Study the drawing (mm; zero at the part's minimum x, y, z) and answer. A direction names the side the tool comes from. Coordinates: 2 decimals unless noted, no trailing zeros. Loops run counter-clockwise (first coordinate to the right, second up) from the corner with the lowest first, then second, coordinate; pieces in that order, holes last. Notation, with made-up numbers: (80.5, 35.5) -> (106.5, 35.5) arc R32 ccw to (106.5, 70.5) -> close; hole circle Ø1 at (68, 37). An arc over 180 degrees is marked (long way). Answer as a JSON object with one key per item and string values. Group by question number.
Q1. The part is cut by section B-B on z = 4.75. Write down the section's boundary in (x, y) (1 decimal).
Q2. Determine the mould class of the marked faces 1, 2 and 3 for opening direction X: released by +X, released by -X, zero draft, split by the parting line, or undercut.
Q3. For the marked faces 4, 5 and 6, determine the directions among +Z, -Z, +X, -X, +Y, -Y from which every point of the face is accessible in a straight line to the end or side of a thin tool.
Q4. The part is cut by section C-C on x = 18. Write down the section's boundary in (y, z).
Q5. Straight lines are drawn through the part: line 1 along X through (y, z) = (1.25, 3.5); line 2 along Y through (x, z) = (18.5, 3.5); line 3 along X through (y, z) = (13, 3.5) (1 decimal). For each, find the intervals that lie inside material, in ascending order. Write a range as [from, to].
Q6. The part is cut by section D-D on y = 9.5. Write down the section's boundary in (x, z) (1 decimal).
Q7. The part is cut by section A-A on y = 6.25. Write down the section's boundary in (x, z) (1 decimal).
Q8. Each of these flat-tipped pins is pushed along its axis until it touches: P1, Ø5.5, axis at x = 18.5, z = 6, coming from the -Y side; P2, Ø4, axis at y = 7, z = 5, coming from the +X side; P3, Ø2.5, axis at x = 3.5, z = 9.5, coming from the +Y side. Where does it stop, or does it pass through?
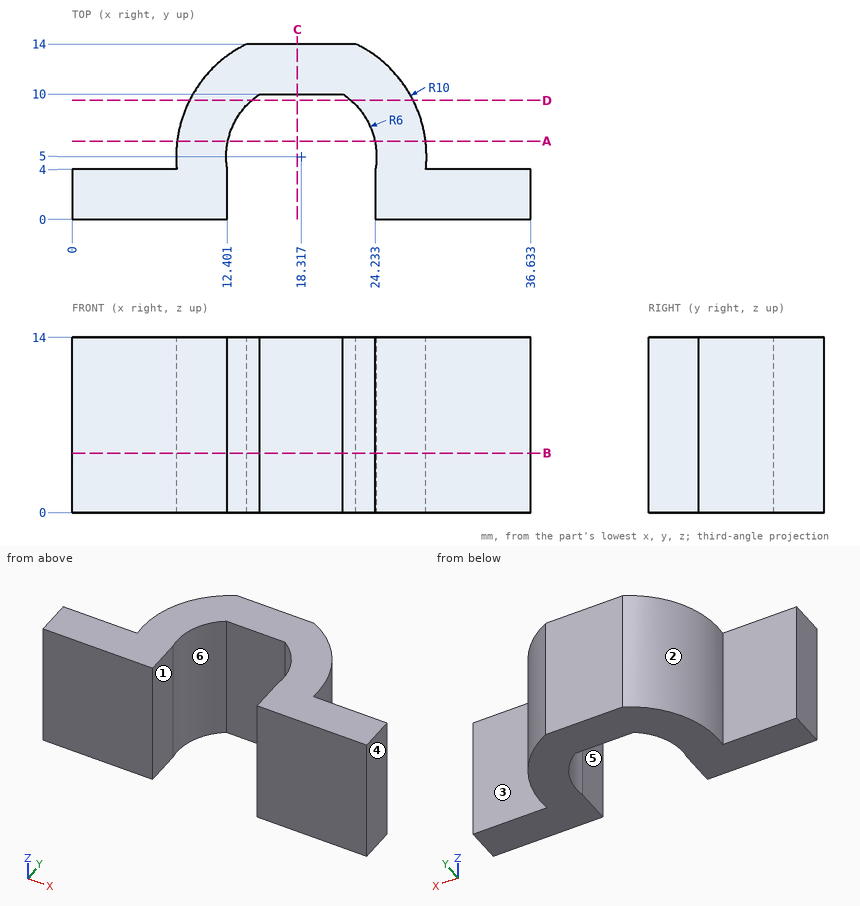
Final values:
{
 "1": {"outline": "(0, 0) -> (12.4, 0) -> (12.4, 4) arc R6 cw to (15, 10) -> (21.6, 10) arc R6 cw to (24.2, 4) -> (24.2, 0) -> (36.6, 0) -> (36.6, 4) -> (28.3, 4) arc R10 ccw to (22.7, 14) -> (14, 14) arc R10 ccw to (8.4, 4) -> (0, 4) -> close"},
 "2": {"face 1": "undercut", "face 2": "released by -X", "face 3": "zero draft"},
 "3": {"face 4": "+Z, -Z, +X, +Y, -Y", "face 5": "+Z, -Z, -Y", "face 6": "+Z, -Z"},
 "4": {"outline": "(10, 0) -> (14, 0) -> (14, 14) -> (10, 14) -> close"},
 "5": {"line 1": "x = [0, 12.4], [24.23, 36.63]", "line 2": "y = [10, 14]", "line 3": "x = [12.3, 24.3]"},
 "6": {"outline": "(9.4, 0) -> (14.3, 0) -> (14.3, 14) -> (9.4, 14) -> close; (22.3, 0) -> (27.2, 0) -> (27.2, 14) -> (22.3, 14) -> close"},
 "7": {"outline": "(8.4, 0) -> (12.4, 0) -> (12.4, 14) -> (8.4, 14) -> close; (24.2, 0) -> (28.2, 0) -> (28.2, 14) -> (24.2, 14) -> close"},
 "8": {"P1": "stops at y = 10", "P2": "stops at x = 28.32", "P3": "stops at y = 4"}
}
